Autodesk Inventor part; units mm, degrees
ref_plane "YZ Plane" through (0, 0, 0) normal (1, 0, 0) x (0, 1, 0)
ref_plane "XZ Plane" through (0, 0, 0) normal (0, 1, 0) x (-1, 0, 0)
ref_plane "XY Plane" through (0, 0, 0) normal (0, 0, 1) x (1, 0, 0)
sketch "Esquisse1" plane through (0, 0, 0) normal (0, 1, 0) x (-1, 0, 0)
  line L0 (0, 0) -> (14, 0)
  line L1 (14, 0) -> (14, -30)
  line L2 (14, -30) -> (0, -30)
  line L3 (0, -30) -> (0, 0)
  line L4 (2, 0) -> (9, 0)
  line L5 (9, 0) -> (9, 3)
  line L6 (9, 3) -> (2, 3)
  line L7 (2, 3) -> (2, 0)
  line L8 (14, -15) -> (0, -15) construction
  line L9 (2, -30) -> (9, -30)
  line L10 (9, -30) -> (9, -33)
  line L11 (9, -33) -> (2, -33)
  line L12 (2, -33) -> (2, -30)
  dimension "d0" = 2
  dimension "d1" = 3
  dimension "d2" = 30
  dimension "d3" = 7
  dimension "d4" = 5
extrude "Plaque1" add sketch "Esquisse1" along normal blind 3
sketch "Esquisse2" plane through (0, 3, 0) normal (0, 1, 0) x (1, 0, 0)
  line L0 (-2, 0) -> (-2, -3) construction
  line L1 (0, 0) -> (-2, 0) construction
  line L2 (0, 30) -> (0, 0) construction
  line L3 (-2, 30) -> (0, 30) construction
  line L4 (-2, 33) -> (-2, 30) construction
  line L5 (-9, 33) -> (-2, 33) construction
  line L6 (-9, 30) -> (-9, 33) construction
  line L7 (-14, 30) -> (-9, 30) construction
  line L8 (-14, 0) -> (-14, 30) construction
  line L9 (-9, 0) -> (-14, 0) construction
  line L10 (-9, -3) -> (-9, 0) construction
  line L11 (-2, -3) -> (-9, -3) construction
  line L12 (-14, 0) -> (-14, 30) construction
  line L13 (-14, 0) -> (-9, 15) construction
  line L14 (-9, 15) -> (-14, 30) construction
  spline S0 degree 2 poles (-14, 0) (-9, 15) (-14, 30) knots 1 1 1 2 2 2
  line L15 (-14, 0) -> (-14, 30)
  line L16 (-9, 15) -> (-14, 15) construction
  line L17 (-14, 0) -> (-14, 30) construction
  dimension "d6" = 5
extrude "Couper1" cut sketch "Esquisse2" against normal blind 3
equation "\"d7\" = Epaisseur"
equation "\"LargeurGrugeage\" = Epaisseur"
equation "\"ProfondeurGrugeage\" = 0.5 * Epaisseur"
equation "\"TailleGrugeage\" = 4 * Epaisseur"
equation "\"RestesMinimum\" = 2 * Epaisseur"
equation "\"Rayondetransition\" = RayonPli"
equation "\"TailleRayonJacobi\" = RayonPli"
equation "\"TailleJeu\" = Epaisseur"
equation "\"d5\" = RayonPli"
properties part number "tip_up" material "Plastique PMMA"
Source: CAD feature listing. Evaluate the final solid. Frame: model axes, mm. A direction names the side the tool comes from. Round coordinates to 2 decimals unless told otherwise and drop trailing zeros. Loops run counter-clockwise (first coordinate to the right, second up) from the corner with the lowest first, then second, coordinate; pieces in that order, holes last. Notation, with made-up numbers: M 88,9 L 112,9 A9 cw 112,23 Z; hole C 31,84 d1. An arc over 180 degrees is marked long. Return JSON: item names as keys, results as strings. Group by question number.
1. Material intervals for line 1 along Z through (x, y) = (-10, 1.7); line 2 along X through (y, z) = (0.5, -8); line 3 along X through (y, z) = (0.6, -1.5) (3 decimals), sorted ascending. Write a range as from..to.
2. Section query A-A on x = -10. Output: boundary loops of the cut face in (y, z), and give its area (3 significant figures).
3. Reachability of faces 1 (the face through (-11, 1, 0)), 2 (the face through (-1, 1, -30)), 3 (the face through (-2, 1, 2)) from +Z, -Z, +X, -X, +Y, -Y: full face, straight path, thin tool, end or side. Return the list, or none.
4. Pin query (flat end, axial travel): pin 1 (1.5 mm diameter, centred on x = -11.5, y = 1, fed in from +Z); pin 2 (1.5 mm diameter, centred on y = 1.5, z = 1.5, fed in from +X); pin 3 (4 mm diameter, centred on x = -1.5, z = -9.5, fed in from -Y). Return the tip coordinate at first contact, or that it passes through.
Checks:
{
 "1": {"line 1": "z = -30..0", "line 2": "x = -12.04..0", "line 3": "x = -13.525..0"},
 "2": {"outline": "M 0,-30 L 3,-30 L 3,0 L 0,0 Z", "area": "90.0 mm²"},
 "3": {"face 1": "+Z, -X, +Y, -Y", "face 2": "-Z, +X, +Y, -Y", "face 3": "+Z, +X, +Y, -Y"},
 "4": {"pin 1": "stops at z = 0", "pin 2": "stops at x = -2", "pin 3": "stops at y = 0"}
}
